```python
from build123d import *

# Parameters (mm, degrees)
F0_W     = 25.4
F0_H     = 19.05
F0_W_2   = 469.9
F0_H_2   = 152.4
F0_W_3   = 111.76
F0_H_3   = 57.15
F1_DEPTH = 19.05


# Not quite as in the source:
# - a feature names something its author has since deleted; it is built from what else it names


with BuildPart() as f1:
    # F0 (on Front) → F1 (new body)
    with BuildSketch(Plane.XZ):
        Polygon((-448.4900477648, 138.0508303034), (-505.6400477648, 138.0508303034), (-505.6400477648, -166.7491696966), (-448.4900477648, -166.7491696966), (-448.4900477648, -147.6991696966), (-359.5900477648, -147.6991696966), (-359.5900477648, -166.7491696966), (-232.5900477648, -166.7491696966), (-232.5900477648, -147.6991696966), (-143.6900477648, -147.6991696966), (-143.6900477648, -166.7491696966), (-16.6900477648, -166.7491696966), (-16.6900477648, -147.6991696966), (72.2099522352, -147.6991696966), (72.2099522352, -166.7491696966), (542.1099522352, -166.7491696966), (542.1099522352, -49.2741696966), (523.0599522352, -49.2741696966), (497.6599522352, -49.2741696966), (474.7999522352, -49.2741696966), (449.3999522352, -49.2741696966), (430.3499522352, -49.2741696966), (430.3499522352, -23.8741696966), (430.3499522352, 20.5758303034), (430.3499522352, 77.7258303034), (430.3499522352, 90.4258303034), (430.3499522352, 128.5258303034), (449.3999522352, 128.5258303034), (474.7999522352, 128.5258303034), (497.6599522352, 128.5258303034), (523.0599522352, 128.5258303034), (542.1099522352, 128.5258303034), (542.1099522352, 138.0508303034), (474.7999522352, 138.0508303034), (449.3999522352, 138.0508303034), (72.2099522352, 138.0508303034), (72.2099522352, 119.0008303034), (-16.6900477648, 119.0008303034), (-16.6900477648, 138.0508303034), (-143.6900477648, 138.0508303034), (-143.6900477648, 119.0008303034), (-232.5900477648, 119.0008303034), (-232.5900477648, 138.0508303034), (-359.5900477648, 138.0508303034), (-359.5900477648, 119.0008303034), (-448.4900477648, 119.0008303034), align=None)
        with Locations((462.0999522352, -77.8491696966)):
            Rectangle(F0_W, F0_H, mode=Mode.SUBTRACT)
        with Locations((510.3599522352, -77.8491696966)):
            Rectangle(F0_W, F0_H, mode=Mode.SUBTRACT)
        with Locations((307.1599522352, -242.9491696966)):
            Rectangle(F0_W_2, F0_H_2)
        Polygon((72.2099522352, 290.4508303034), (72.2099522352, 138.0508303034), (449.3999522352, 138.0508303034), (474.7999522352, 138.0508303034), (542.1099522352, 138.0508303034), (542.1099522352, 290.4508303034), align=None)
        with Locations((462.0999522352, 157.1008303034)):
            Rectangle(F0_W, F0_H, mode=Mode.SUBTRACT)
        with Locations((510.3599522352, 157.1008303034)):
            Rectangle(F0_W, F0_H, mode=Mode.SUBTRACT)
        with Locations((486.2299522352, 49.1508303034)):
            Rectangle(F0_W_3, F0_H_3)
        with Locations((462.0999522352, 49.1508303034)):
            Rectangle(F0_W, F0_H, mode=Mode.SUBTRACT)
        with Locations((510.3599522352, 49.1508303034)):
            Rectangle(F0_W, F0_H, mode=Mode.SUBTRACT)
    extrude(amount=F1_DEPTH)


solid = f1.part
```
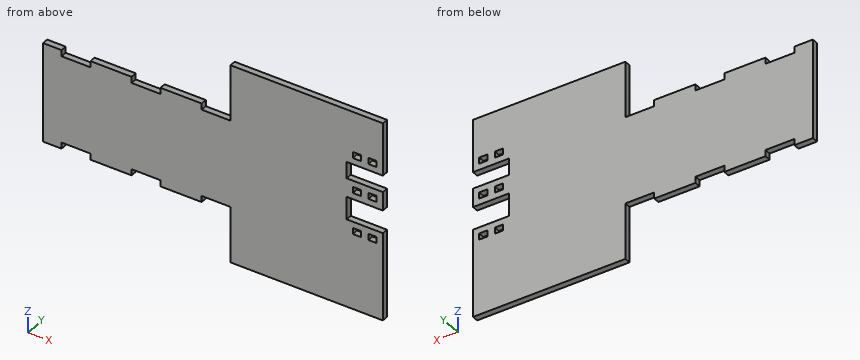
Build history of the part. All positions in model axes, mm. Round coordinates to 2 decimals unless told otherwise and drop trailing zeros. Loops run counter-clockwise (first coordinate to the right, second up) from the corner with the lowest first, then second, coordinate; pieces in that order, holes last.
Item 1: Saw through at A-A (y = -3.5). State how many separate pieces and enclosed holes the cut face has, then the cut area to 3 significant figures.
Item 2: Saw through at B-B (x = -332.5). List the corners of the cut face in (y, z).
Item 3: Pin check, flat tips, straight feed: P1, Ø9.5, axis at x = -174, y = -5, coming from the +Z side; P2, Ø4, axis at x = -261.5, y = -11.5, coming from the -Z side. Stop position of each tip, or through.
Item 4: Drill centre lines: line 1 along X through (y, z) = (-16.5, -68.5); line 2 along X through (y, z) = (-4, 166); line 3 along X through (y, z) = (-3.5, -156.5). Where is each one in solid material? Low to high.
Item 5: Saw through at C-C (z = -266.5). List the corners of the cut face in (x, y), then the cut area to 3 significant figures.
Worked answers:
1. separate pieces: 1
1. enclosed holes: 6
1. area: 436,000 mm2
2. outline: (-19.05, -166.75) - (0, -166.75) - (0, 138.05) - (-19.05, 138.05) - close
3. P1: stops at z = 119
3. P2: stops at z = -166.75
4. line 1: x = -505.64 to 449.4, 474.8 to 497.66, 523.06 to 542.11
4. line 2: x = 72.21 to 449.4, 474.8 to 497.66, 523.06 to 542.11
4. line 3: x = -505.64 to -448.49, -359.59 to -232.59, -143.69 to -16.69, 72.21 to 542.11
5. outline: (72.21, -19.05) - (542.11, -19.05) - (542.11, 0) - (72.21, 0) - close
5. area: 8,950 mm2
